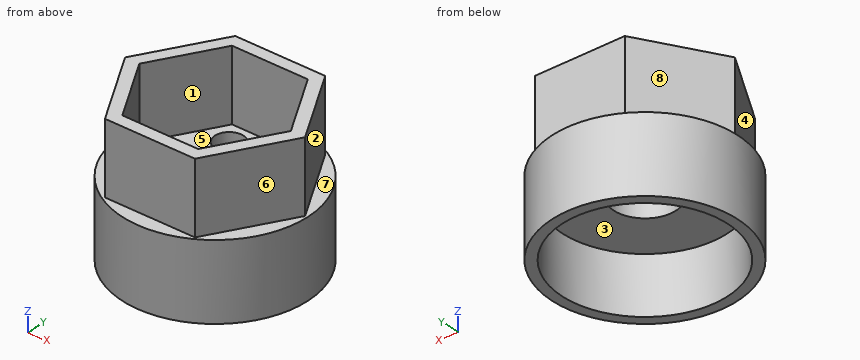
from build123d import *

# Parameters (mm, degrees)
F2_DEPTH  = 19.05
F3_DEPTH  = 67.818
F4_R      = 24.7218142408
F5_DEPTH  = 2.54
F6_R      = 8.255
F7_DEPTH  = 60.706
F8_DEPTH  = 17.78
F9_R      = 22.0208797998
F9_R_2    = 8.255
F10_DEPTH = 15.24
F11_R     = 3.81
F12_DEPTH = 25.4


with BuildPart() as f2:
    # F0 (on Top) → F2 (new body)
    with BuildSketch(Plane.XY):
        Polygon((11.9120152821, -20.8982058203), (24.0543847749, -0.1329950655), (12.1423694928, 20.7652107547), (-11.9120152821, 20.8982058203), (-24.0543847749, 0.1329950655), (-12.1423694928, -20.7652107547), align=None)
    extrude(amount=F2_DEPTH)

    # F1 (on face) → F3 (cut)
    with BuildSketch(Plane.XY):
        Polygon((20.2553256916, -0.1120183326), (10.2246735675, 17.4856174446), (-10.0306521241, 17.5976357771), (-20.2553256916, 0.1120183326), (-10.2246735675, -17.4856174446), (10.0306521241, -17.5976357771), align=None)
    extrude(amount=F3_DEPTH, mode=Mode.SUBTRACT)

    # F4 (on Top) → F5 (join)
    with BuildSketch(Plane.XY):
        Circle(F4_R)
    extrude(amount=-F5_DEPTH)

    # F6 (on face) → F7 (cut)
    with BuildSketch(Plane.XY):
        Circle(F6_R)
    extrude(amount=-F7_DEPTH, mode=Mode.SUBTRACT)

    # F8 (add): a face of the model
    f8_faces = [f2.faces().sort_by_distance(p)[0] for p in [
        (-24.0225757411, 0, -2.54),
    ]]
    extrude(f8_faces, amount=F8_DEPTH)

    # F9 (on face) → F10 (cut)
    with BuildSketch(Plane(origin=(0, 0, -20.32), x_dir=(1, 0, 0), z_dir=(0, 0, -1))):
        Circle(F9_R)
        Circle(F9_R_2, mode=Mode.SUBTRACT)
    extrude(amount=-F10_DEPTH, mode=Mode.SUBTRACT)

    # F11 (on face) → F12 (cut)
    with BuildSketch(Plane.XY):
        with Locations((-6.1764977872, 12.0172752067)):
            Circle(F11_R)
    extrude(amount=-F12_DEPTH, mode=Mode.SUBTRACT)


solid = f2.part
Geometry check sheet. Reference: the model listing, model coordinates, mm. Face numbers are marked on the shaded views. A direction names the side the tool comes from. Round coordinates to 2 decimals unless told otherwise and drop trailing zeros. Write each loop counter-clockwise with the first axis right and the second up, starting at its lowest first coordinate (ties: lowest second). Pieces come first, ordered by that corner, then holes.
Item 1: Section check D-D (y = -20). Record the boundary of the cut face in (x, z), plus the area to 3 significant figures.
Determined:
outline: (-14.53, -20.32) - (-9.22, -20.32) - (-9.22, -5.08) - (9.22, -5.08) - (9.22, -20.32) - (14.53, -20.32) - (14.53, 0) - (12.44, 0) - (12.44, 19.05) - (-12.58, 19.05) - (-12.58, 0) - (-14.53, 0) - close
area: 786 mm2
Item 2: Section check B-B (z = 16.5). Record the boundary of the cut face in (x, y), plus the area to 3 significant figures.
Determined:
outline: (-24.05, 0.13) - (-12.14, -20.77) - (11.91, -20.9) - (24.05, -0.13) - (12.14, 20.77) - (-11.91, 20.9) - close; hole (-20.26, 0.11) - (-10.22, -17.49) - (10.03, -17.6) - (20.26, -0.11) - (10.22, 17.49) - (-10.03, 17.6) - close
area: 437 mm2
Item 3: Material ranges on line 1 along X through (y, z) = (0.5, -17); line 2 along Y through (x, z) = (0, -3.8) (3 decimals); line 3 along X through (y, z) = (-11, -7), recorded low to high.
Determined:
line 1: x = -24.72 to -22.02, 22.02 to 24.72
line 2: y = -24.722 to -8.255, 8.255 to 24.722
line 3: x = -22.14 to -19.08, 19.08 to 22.14
Item 4: Section check C-C (x = 0). Record the boundary of the cut face in (y, z) (3 decimals), plus the area to 3 significant figures.
Determined:
outline: (-24.722, -20.32) - (-22.021, -20.32) - (-22.021, -5.08) - (-8.255, -5.08) - (-8.255, 0) - (-17.542, 0) - (-17.542, 19.05) - (-20.832, 19.05) - (-20.832, 0) - (-24.722, 0) - close; (8.255, -5.08) - (22.021, -5.08) - (22.021, -20.32) - (24.722, -20.32) - (24.722, 0) - (20.832, 0) - (20.832, 19.05) - (17.542, 19.05) - (17.542, 0) - (8.255, 0) - close
area: 375 mm2
Item 5: Mould release check, pull along Y, two halves, no side actions. Record for the marked faces 5, 6, 7 and 8: +Y half, -Y half, draft (parallel to the pull), parting line (faces both ways), or undercut.
Determined:
face 5: undercut
face 6: -Y half
face 7: draft
face 8: +Y half
Item 6: Go/stop test with flat-tipped pins: pin 1 Ø12 at (x, y) = (1.5, -11.5) entering from -Z; pin 2 Ø1 at (x, z) = (14.5, 0) entering from +Y; pin 3 Ø10 at (x, z) = (1.5, -6) entering from +Y. Record where each tip stops, or that it passes through.
Determined:
pin 1: stops at z = -5.08
pin 2: stops at y = 20.38
pin 3: stops at y = 24.72
Item 7: Access from +Z, -Z, +X, -X, +Y, -Y to the whole of each face (thin tool, end or side, straight path). Record for the marked faces 1, 2, 3 and 4.
Determined:
face 1: +Z
face 2: +Z, +X, +Y
face 3: -Z
face 4: +Z, -X, -Y
Item 8: Section check A-A (y = -5). Record the boundary of the cut face in (x, z).
Determined:
outline: (-24.21, -20.32) - (-21.45, -20.32) - (-21.45, -5.08) - (-6.57, -5.08) - (-6.57, 0) - (-17.34, 0) - (-17.34, 19.05) - (-21.13, 19.05) - (-21.13, 0) - (-24.21, 0) - close; (6.57, -5.08) - (21.45, -5.08) - (21.45, -20.32) - (24.21, -20.32) - (24.21, 0) - (21.21, 0) - (21.21, 19.05) - (17.4, 19.05) - (17.4, 0) - (6.57, 0) - close
